Source: CAD feature listing. Evaluate the final solid. Frame: model axes, mm. A direction names the side the tool comes from. Round coordinates to 2 decimals unless told otherwise and drop trailing zeros. Order: outer loops, then holes, each group sorted by start corner. A loop starts at its lowest first (then second) coordinate and runs counter-clockwise, first axis right, second up. Notation, with made-up numbers: M -14.75,-32 L 21.25,-32 A12 ccw 21.25,-21 Z; hole C -31.75,63 d8. An arc over 180 degrees is marked long. Use CSV: the item, a comma, the result in double quotes. Start each with the question number.
```python
from build123d import *

# Parameters (mm, degrees)
F0_W      = 9.5
F0_H      = 10
F1_DEPTH  = 9.5
F3_DEPTH  = 9.5
F8_SIZE   = 1.99999
F10_D     = 2.8
F10_DEPTH = 5
F10_TIP   = 0.8412048666
F11_R     = 0.5


# Not quite as in the source:
# - a fillet or chamfer is up to 0.001 mm smaller than in the source, because OpenCascade refuses the exact size


with BuildPart() as f1:
    # F0 (on Front) → F1 (new body)
    with BuildSketch(Plane.XZ):
        with Locations((4.75, 5)):
            Rectangle(F0_W, F0_H)
    extrude(amount=F1_DEPTH)

    # F2 (on Front) → F3 (join)
    with BuildSketch(Plane.XZ):
        Polygon((7.5, 10), (9.5, 10), (9.5, 34), (5, 34), (5, 32), (7.5, 32), align=None)
    extrude(amount=F3_DEPTH)


with BuildPart() as f5_1:
    # F5: instance of F1
    add(f1.part.mirror(Plane(origin=(4.75, -4.75, 5), x_dir=(0, -1, 0), z_dir=(-1, 0, 0))))


with BuildPart() as f1_1:
    add(f1.part)

    # F6: union 

    # F7: union F5_1
    add(f5_1.part)

    # F8 (size 2 in the source; OpenCascade refuses exactly that, so slightly less here)
    f8_edges = [f1_1.edges().sort_by_distance(p)[0] for p in [
        (9.5, -9.5, 17),
        (9.5, 0, 17),
        (0, -9.5, 17),
        (0, 0, 17),
    ]]
    chamfer(f8_edges, length=F8_SIZE)

    # F10
    with Locations(Plane(origin=(0, 0, 0), x_dir=(1, 0, 0), z_dir=(0, 0, -1))):
        with Locations((4.75, 4.75)):
            Hole(F10_D / 2, depth=F10_DEPTH)
            with Locations((0, 0, -(F10_DEPTH + F10_TIP / 2))):  # 118° drill point
                Cone(0, F10_D / 2, F10_TIP, mode=Mode.SUBTRACT)

    # F11
    f11_edges = [f1_1.edges().sort_by_distance(p)[0] for p in [
        (2, -4.75, 10),
        (7.5, -4.75, 10),
        (2, -4.75, 32),
        (7.5, -4.75, 32),
    ]]
    fillet(f11_edges, radius=F11_R)


solid = f1_1.part
```
(1) Draft query along X for faces 4 (the face through (4.8, -9.5, 9.7)), 5 (the face through (9.5, -5, 17)), 6 (the face through (7.5, -5, 21)). Return one class per face: pulls with the +X half, pulls with the -X half, needs draft (parallel to the pull), parting line crosses it, or undercut.
(2) Reachability of faces 1 (the face through (5, -5, 10)), 2 (the face through (4.5, -5, 33)), 3 (the face through (3.415, -5.171, 2.535)) from +Z, -Z, +X, -X, +Y, -Y: full face, straight path, thin tool, end or side. Return the list, or none.
(3) Line query: line 1 along X through (y, z) = (-7, 23); line 2 along Y through (x, z) = (4.75, 2); line 3 along X through (y, z) = (-4.75, 2.05). Output: solid intervals per line, ascending.
(4) Section B-B on y = -2.75. Return loops of the section in (x, z).
(5) Section C-C on y = -8. Return loops of the section in (x, z).
(6) Contact query for flat-ended pins moving along their axis: P1, Ø1.6, axis at x = 3.5, y = -2.5, coming from the -Z side; P2, Ø1.5, axis at x = 5, z = 21, coming from the +Y side; P3, Ø5, axis at x = 8, z = 25, coming from the -Y side. Output: stop coordinate, or through.
Results below:
1,face 4,"needs draft"
1,face 5,"pulls with the +X half"
1,face 6,"undercut"
2,face 1,"+Y, -Y"
2,face 2,"+Z, +Y, -Y"
2,face 3,"-Z"
3,line 1,"x = 0 to 2, 7.5 to 9.5"
3,line 2,"y = -9.5 to -6.15, -3.35 to 0"
3,line 3,"x = 0 to 3.35, 6.15 to 9.5"
4,outline,"M 0,0 L 9.5,0 L 9.5,34 L 5,34 L 5,32 L 7,32 A0.5 cw 7.5,31.5 L 7.5,10.5 A0.5 cw 7,10 L 2.5,10 A0.5 cw 2,10.5 L 2,31.5 A0.5 cw 2.5,32 L 4.5,32 L 4.5,34 L 0,34 Z"
5,outline,"M 0.5,0 L 9,0 L 9,34 L 5,34 L 5,32 L 7,32 A0.5 cw 7.5,31.5 L 7.5,10.5 A0.5 cw 7,10 L 2.5,10 A0.5 cw 2,10.5 L 2,31.5 A0.5 cw 2.5,32 L 4.5,32 L 4.5,34 L 0.5,34 Z"
6,P1,"stops at z = 0"
6,P2,"passes through"
6,P3,"stops at y = -9.5"
